Source: CAD feature listing. Evaluate the final solid. Frame: model axes, mm. A direction names the side the tool comes from. Give positions to 0.01 mm unless a question says otherwise; leave off trailing zeros. Loops run counter-clockwise (first coordinate to the right, second up) from the corner with the lowest first, then second, coordinate; pieces in that order, holes last. Notation, with made-up numbers: (-24, -20) -> (9, -20) arc R26 ccw to (9, 10) -> close; hole circle Ø4 at (71, 22.25). An arc over 180 degrees is marked (long way). Return JSON: item names as keys, results as strings. Group by question number.
(1) Cut plane B-B on x = -0.5. Return loops of the section in (y, z).
(2) Cut plane C-C on y = 2.25. Return loops of the section in (x, z).
(3) Cut plane A-A on z = 4.3. Return loops of the section in (x, y).
(4) Draft query along Y for faces 3 (the face through (0, 3, 0)), 4 (the face through (0, 4.753, 4)), 5 (the face through (0, 0, 3)). Return one class per face: released by +Y, released by -Y, zero draft, split by the parting line, or undercut.
(5) Cut plane D-D on z = 1.7. Return loops of the section in (x, y).
(6) Pin query (flat end, axial travel): pin 1 (3 mm diameter, centred on x = -1.5, y = 2.5, fed in from +Z); pin 2 (0.8 mm diameter, centred on x = -1.5, z = 3.5, fed in from -Y). Return the tip coordinate at first contact, or that it passes through.
(7) Ray query, line 1 (Z direction, x = 3, y = 4.25); line 2 (Y direction, x = -2.5, z = 3.05); line 3 (Y direction, x = 0, z = 2.6). Return the intervals inside material, ascending. Write a range as from..to.
(8) Access query for faces 1 (the face through (0, 1, 5.08)), 2 (the face through (0, 3, 2.54)). Directions: +Z, -Z, +X, -X, +Y, -Y. A direction counts if a zero-diameter tool reaches every point of the face in a straight line with its end or side. Return the directions, or none.
```python
from build123d import *

# Parameters (mm, degrees)
BOSS_EXTRUDE1_DEPTH = 5.08
SKETCH2_W           = 7.112
SKETCH2_H           = 3.556
CUT_EXTRUDE1_DEPTH  = 2.54


with BuildPart() as part:
    # Sketch1 → Boss-Extrude1 (new body)
    with BuildSketch(Plane.XY):
        with BuildLine():
            Line((-3.556, -0.199764438), (-3.556, 6.150235562))
            Line((-3.556, 6.150235562), (3.556, 6.150235562))
            Line((3.556, 6.150235562), (3.556, -0.199764438))
            ThreePointArc((3.556, -0.199764438), (0, 0), (-3.556, -0.199764438))
        make_face()
    extrude(amount=BOSS_EXTRUDE1_DEPTH)

    # Sketch2 → Cut-Extrude1 (cut)
    with BuildSketch(Plane.XY.offset(5.08)):
        with Locations((0, 2.975235562)):
            Rectangle(SKETCH2_W, SKETCH2_H)
    extrude(amount=-CUT_EXTRUDE1_DEPTH, mode=Mode.SUBTRACT)


solid = part.part
```
Answers:
{
 "1": {"outline": "(0, 0) -> (6.15, 0) -> (6.15, 5.08) -> (4.75, 5.08) -> (4.75, 2.54) -> (1.2, 2.54) -> (1.2, 5.08) -> (0, 5.08) -> close"},
 "2": {"outline": "(-3.56, 0) -> (3.56, 0) -> (3.56, 2.54) -> (-3.56, 2.54) -> close"},
 "3": {"outline": "(-3.56, -0.2) arc R31.75 cw to (3.56, -0.2) -> (3.56, 1.2) -> (-3.56, 1.2) -> close; (-3.56, 4.75) -> (3.56, 4.75) -> (3.56, 6.15) -> (-3.56, 6.15) -> close"},
 "4": {"face 3": "zero draft", "face 4": "undercut", "face 5": "released by -Y"},
 "5": {"outline": "(-3.56, -0.2) arc R31.75 cw to (3.56, -0.2) -> (3.56, 6.15) -> (-3.56, 6.15) -> close"},
 "6": {"pin 1": "z = 5.08", "pin 2": "y = -0.06"},
 "7": {"line 1": "0..2.54", "line 2": "-0.1..1.2, 4.75..6.15", "line 3": "0..1.2, 4.75..6.15"},
 "8": {"face 1": "+Z, +X, -X, +Y, -Y", "face 2": "+Z, +X, -X"}
}
